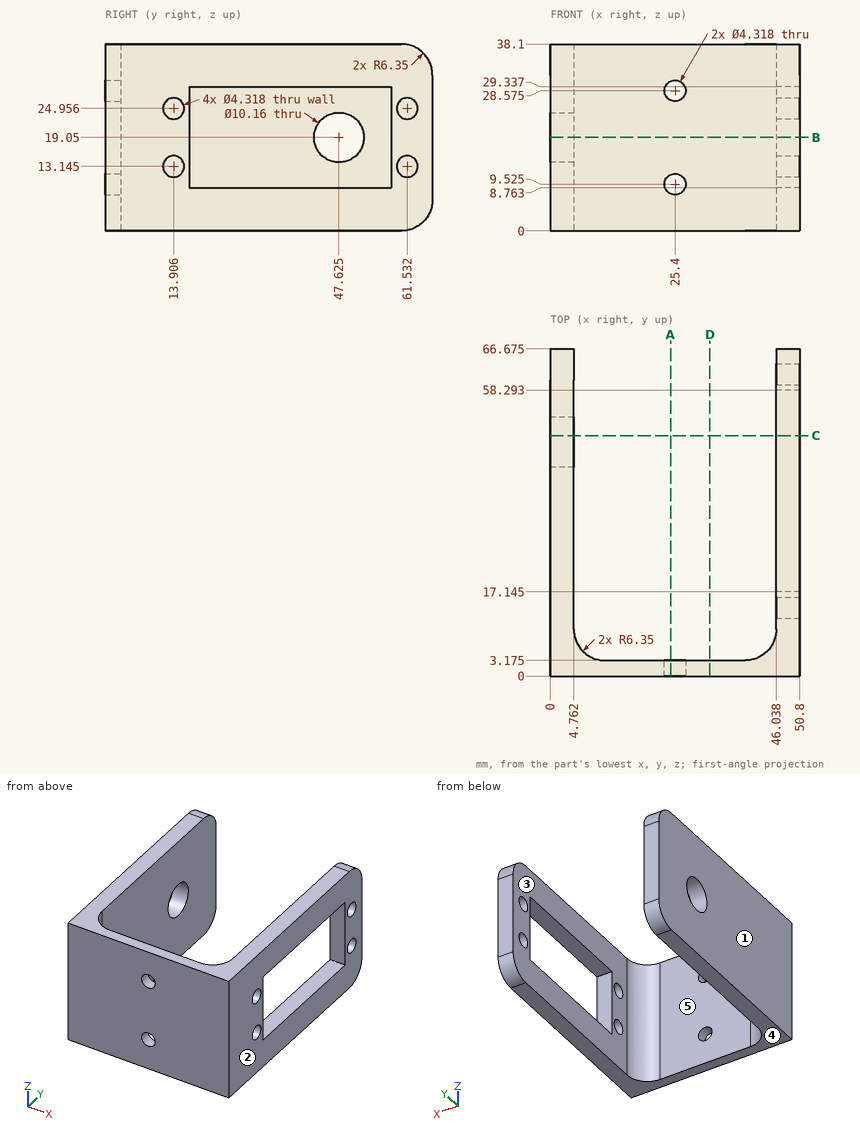
Geometry check sheet. Reference: drawing and pictorial views, mm from the part's lowest x, y, z. A direction names the side the tool comes from. Coordinates: 2 decimals unless noted, no trailing zeros. Order: outer loops, then holes, each group sorted by start corner. A loop starts at its lowest first (then second) coordinate and runs counter-clockwise, first axis right, second up.
Item 1: Section check D-D, the plane x = 32.5. Enter the section's corners in (y, z) (1 decimal).
Filled in:
outline: (0, 0) - (3.2, 0) - (3.2, 38.1) - (0, 38.1) - close
Item 2: Section check A-A, the plane x = 24.5. Enter the section's corners in (y, z) (1 decimal).
Filled in:
outline: (0, 0) - (3.2, 0) - (3.2, 7.6) - (0, 7.6) - close; (0, 11.5) - (3.2, 11.5) - (3.2, 26.6) - (0, 26.6) - close; (0, 30.5) - (3.2, 30.5) - (3.2, 38.1) - (0, 38.1) - close
Item 3: Section check C-C, the plane y = 49. Enter the section's corners in (x, z).
Filled in:
outline: (0, 0) - (4.76, 0) - (4.76, 14.16) - (0, 14.16) - close; (0, 23.94) - (4.76, 23.94) - (4.76, 38.1) - (0, 38.1) - close; (46.04, 0) - (50.8, 0) - (50.8, 8.76) - (46.04, 8.76) - close; (46.04, 29.34) - (50.8, 29.34) - (50.8, 38.1) - (46.04, 38.1) - close
Item 4: Material ranges on L1, parallel to X at y = 34, z = 8.5; L2, parallel to X at y = 42.5, z = 27; L3, parallel to Y at x = 17, z = 19 (1 decimal), recorded low to high.
Filled in:
L1: x = 0 to 4.76, 46.04 to 50.8
L2: x = 0 to 4.76
L3: y = 0 to 3.2
Item 5: Access from +Z, -Z, +X, -X, +Y, -Y to the whole of each face (thin tool, end or side, straight path). Record for the marked faces 4 and 5.
Filled in:
face 4: -Z, +X, -X, +Y, -Y
face 5: +Z, -Z, +Y
Item 6: Section check B-B, the plane z = 19.05. Give the number of separate pieces and of enclosed holes in the cut face, then the cut area to 3 significant figures.
Filled in:
separate pieces: 3
enclosed holes: 0
area: 539 mm2
Item 7: Depth check by flat-ended pin: pin 1 (7 mm diameter, centred on y = 13.91, z = 24.96, fed in from -X); pin 2 (1.5 mm diameter, centred on x = 10.5, z = 22, fed in from +Y); pin 3 (1.5 mm diameter, centred on x = 26, z = 28.5, fed in from -Y). Enter the tip coordinate at first touch or a pass-through.
Filled in:
pin 1: stops at x = 0
pin 2: stops at y = 3.32
pin 3: passes through
Item 8: Release check for a two-part mould opening along X. For the marked faces 1, 2 and 3 record: +X half, -X half, draft (parallel to the pull), parting line (faces both ways), or undercut.
Filled in:
face 1: -X half
face 2: +X half
face 3: undercut
